Check sheet for the modelled part. Datum: model origin and axes. Units: mm. Round coordinates to 2 decimals unless told otherwise and drop trailing zeros. Order: outer loops, then holes, each group sorted by start corner. A loop starts at its lowest first (then second) coordinate and runs counter-clockwise, first axis right, second up. Notation, with made-up numbers: (71, 15) -> (95, 15) arc R10 cw to (95, 28) -> close; hole circle Ø1 at (31, -5.75). An arc over 180 degrees is marked (long way). Answer in a Markdown table with one row per item.
from build123d import *

# Parameters (mm, degrees)
EXTRUDE1_DEPTH = 0.5
FILLET1_R      = 3
SKETCH3_R      = 13.5
SKETCH3_R_2    = 3.5
SKETCH3_R_3    = 6.25
EXTRUDE2_DEPTH = 0.5
FILLET2_R      = 1


with BuildPart() as part:
    # Sketch1 → Revolve1 (revolve)
    with BuildSketch(Plane(origin=(0, 0, 0), x_dir=(0, 0, -1), z_dir=(1, 0, 0))):
        with BuildLine():
            Line((40, 36), (41.424630354, 28))
            ThreePointArc((41.424630354, 28), (44.158804332, -23.452078799), (0, -50))
            Line((0, -50), (0, 36))
            Line((0, 36), (40, 36))
        make_face()
    revolve(axis=Axis((0, 36, 0), (0, -1, 0)))

    # Sketch2 → Extrude1 (cut)
    with BuildSketch(Plane(origin=(0, 36, 0), x_dir=(1, 0, 0), z_dir=(0, 1, 0))):
        with BuildLine():
            Line((17.811513131, 33), (-17.811513131, 33))
            ThreePointArc((-17.811513131, 33), (-37.5, 0), (-17.811513131, -33))
            Line((-17.811513131, -33), (17.811513131, -33))
            ThreePointArc((17.811513131, -33), (32.20389528, -19.213514223), (37.5, 0))
            ThreePointArc((37.5, 0), (32.20389528, 19.213514223), (17.811513131, 33))
        make_face()
    extrude(amount=-EXTRUDE1_DEPTH, mode=Mode.SUBTRACT)

    # Fillet1
    # the kernel refuses this fillet: 3 mm, written as the material it adds along each edge
    with BuildSketch(Plane(origin=(-21.957294119, 35.5, 33), x_dir=(0, 1.0, -3.3253400033406348e-12), z_dir=(1, 0, 0)), Plane(origin=(21.957294119, 35.5, -33), x_dir=(0, 1.0, 3.3253400033406348e-12), z_dir=(-1, 0, 0))) as fillet1_piece_1:
        with BuildLine():
            CenterArc((3, -1.658312395), FILLET1_R, 146.442690238, 33.557309762)
            Line((0, -1.658312395), (0, 0))
            Line((0, 0), (0.5, 0))
        make_face()
    extrude(amount=43.914588237)
    with BuildSketch(Plane(origin=(0, 35.5, 0), x_dir=(0.37490714563861727, 0, 0.9270623669144945), z_dir=(-0.9270623669144945, 0, 0.37490714563861727))) as fillet1_piece_2:
        with BuildLine():
            CenterArc((35.841687605, 3), FILLET1_R, 270, 33.557309762)
            Line((35.841687605, 0), (37.5, 0))
            Line((37.5, 0), (37.5, 0.5))
        make_face()
    revolve(axis=Axis((0, 35.5, 0), (0, 1, 0)), revolution_arc=135.962852024)
    with BuildSketch(Plane(origin=(0, 35.5, 0), x_dir=(-0.37490714563861693, 0, -0.9270623669144946), z_dir=(0.9270623669144946, 0, -0.37490714563861693))) as fillet1_piece_3:
        with BuildLine():
            CenterArc((35.841687605, 3), FILLET1_R, 270, 33.557309762)
            Line((35.841687605, 0), (37.5, 0))
            Line((37.5, 0), (37.5, 0.5))
        make_face()
    revolve(axis=Axis((0, 35.5, 0), (0, 1, 0)), revolution_arc=135.962852024)

    # Sketch3 → Extrude2 (cut)
    # profile 1 of 10: a face of its own
    with BuildSketch(Plane(origin=(0, 35.5, 0), x_dir=(1, 0, 0), z_dir=(0, 1, 0))):
        with Locations(Location((-17.5, 1.2, 0), (0, 0, 270))):
            Circle(SKETCH3_R)
    # profile 2 of 10: a face of its own
    with BuildSketch(Plane(origin=(0, 35.5, 0), x_dir=(1, 0, 0), z_dir=(0, 1, 0))):
        with Locations(Location((17.5, 1.2, 0), (0, 0, 270))):
            Circle(SKETCH3_R)
        with Locations(Location((17.5, 1.2, 0), (0, 0, 270))):
            Circle(SKETCH3_R_2, mode=Mode.SUBTRACT)
    # profile 3 of 10: a face of its own
    with BuildSketch(Plane(origin=(0, 35.5, 0), x_dir=(1, 0, 0), z_dir=(0, 1, 0))):
        with Locations(Location((0, -20, 0), (0, 0, 270))):
            Circle(SKETCH3_R_3)
    # profile 4 of 10: a face of its own
    with BuildSketch(Plane(origin=(0, 35.5, 0), x_dir=(1, 0, 0), z_dir=(0, 1, 0))):
        with BuildLine():
            Line((-3.75, 24.8), (-1.75, 24.8))
            ThreePointArc((-1.75, 24.8), (-0.75, 23.8), (-1.75, 22.8))
            Line((-1.75, 22.8), (-3.75, 22.8))
            ThreePointArc((-3.75, 22.8), (-4.75, 23.8), (-3.75, 24.8))
        make_face()
    # profile 5 of 10: a face of its own
    with BuildSketch(Plane(origin=(0, 35.5, 0), x_dir=(1, 0, 0), z_dir=(0, 1, 0))):
        with BuildLine():
            Line((-6.5, 27.3), (-4.5, 27.3))
            ThreePointArc((-4.5, 27.3), (-3.5, 26.3), (-4.5, 25.3))
            Line((-4.5, 25.3), (-6.5, 25.3))
            ThreePointArc((-6.5, 25.3), (-7.5, 26.3), (-6.5, 27.3))
        make_face()
    # profile 6 of 10: a face of its own
    with BuildSketch(Plane(origin=(0, 35.5, 0), x_dir=(1, 0, 0), z_dir=(0, 1, 0))):
        with BuildLine():
            Line((-1, 27.3), (1, 27.3))
            ThreePointArc((1, 27.3), (2, 26.3), (1, 25.3))
            Line((1, 25.3), (-1, 25.3))
            ThreePointArc((-1, 25.3), (-2, 26.3), (-1, 27.3))
        make_face()
    # profile 7 of 10: a face of its own
    with BuildSketch(Plane(origin=(0, 35.5, 0), x_dir=(1, 0, 0), z_dir=(0, 1, 0))):
        with BuildLine():
            Line((-3.75, 29.8), (-1.75, 29.8))
            ThreePointArc((-1.75, 29.8), (-0.75, 28.8), (-1.75, 27.8))
            Line((-1.75, 27.8), (-3.75, 27.8))
            ThreePointArc((-3.75, 27.8), (-4.75, 28.8), (-3.75, 29.8))
        make_face()
    # profile 8 of 10: a face of its own
    with BuildSketch(Plane(origin=(0, 35.5, 0), x_dir=(1, 0, 0), z_dir=(0, 1, 0))):
        with BuildLine():
            Line((1.75, 29.8), (3.75, 29.8))
            ThreePointArc((3.75, 29.8), (4.75, 28.8), (3.75, 27.8))
            Line((3.75, 27.8), (1.75, 27.8))
            ThreePointArc((1.75, 27.8), (0.75, 28.8), (1.75, 29.8))
        make_face()
    # profile 9 of 10: a face of its own
    with BuildSketch(Plane(origin=(0, 35.5, 0), x_dir=(1, 0, 0), z_dir=(0, 1, 0))):
        with BuildLine():
            Line((4.5, 27.3), (6.5, 27.3))
            ThreePointArc((6.5, 27.3), (7.5, 26.3), (6.5, 25.3))
            Line((6.5, 25.3), (4.5, 25.3))
            ThreePointArc((4.5, 25.3), (3.5, 26.3), (4.5, 27.3))
        make_face()
    # profile 10 of 10: a face of its own
    with BuildSketch(Plane(origin=(0, 35.5, 0), x_dir=(1, 0, 0), z_dir=(0, 1, 0))):
        with BuildLine():
            Line((1.75, 24.8), (3.75, 24.8))
            ThreePointArc((3.75, 24.8), (4.75, 23.8), (3.75, 22.8))
            Line((3.75, 22.8), (1.75, 22.8))
            ThreePointArc((1.75, 22.8), (0.75, 23.8), (1.75, 24.8))
        make_face()
    extrude(amount=-EXTRUDE2_DEPTH, mode=Mode.SUBTRACT)

    # Fillet2
    # the kernel refuses this fillet: 1 mm, written as the material it adds along each edge
    with BuildSketch(Plane(origin=(0, 35, 20), x_dir=(0, 0, 1), z_dir=(-1, 0, 0))) as fillet2_piece_1:
        with BuildLine():
            CenterArc((5.383974596, 1), FILLET2_R, 270, 60)
            Line((5.383974596, 0), (5.383974596, -0.02))
            Line((5.383974596, -0.02), (6.25, -0.02))
            Line((6.25, -0.02), (6.27, 0))
            ThreePointArc((6.27, 0), (6.27, 0.25), (6.267320508, 0.49))
            Line((6.267320508, 0.49), (6.25, 0.5))
        make_face()
    revolve(axis=Axis((0, 35, 20), (0, 1, 0)))
    with BuildSketch(Plane(origin=(17.5, 35, -1.2), x_dir=(0, 0, 1), z_dir=(-1, 0, 0))) as fillet2_piece_2:
        with BuildLine():
            CenterArc((12.633974596, 1), FILLET2_R, 270, 60)
            Line((12.633974596, 0), (12.633974596, -0.02))
            Line((12.633974596, -0.02), (13.5, -0.02))
            Line((13.5, -0.02), (13.52, 0))
            ThreePointArc((13.52, 0), (13.52, 0.25), (13.517320508, 0.49))
            Line((13.517320508, 0.49), (13.5, 0.5))
        make_face()
    revolve(axis=Axis((17.5, 35, -1.2), (0, 1, 0)))
    with BuildSketch(Plane(origin=(17.5, 35, -1.2), x_dir=(0, 0, 1), z_dir=(-1, 0, 0))) as fillet2_piece_3:
        with BuildLine():
            CenterArc((4.366025404, 1), FILLET2_R, 210, 60)
            Line((3.5, 0.5), (3.482679492, 0.49))
            ThreePointArc((3.482679492, 0.49), (3.48, 0.25), (3.48, 0))
            Line((3.48, 0), (3.5, -0.02))
            Line((3.5, -0.02), (4.366025404, -0.02))
            Line((4.366025404, -0.02), (4.366025404, 0))
        make_face()
    revolve(axis=Axis((17.5, 35, -1.2), (0, 1, 0)))
    with BuildSketch(Plane(origin=(-17.5, 35, -1.2), x_dir=(0, 0, 1), z_dir=(-1, 0, 0))) as fillet2_piece_4:
        with BuildLine():
            CenterArc((12.633974596, 1), FILLET2_R, 270, 60)
            Line((12.633974596, 0), (12.633974596, -0.02))
            Line((12.633974596, -0.02), (13.5, -0.02))
            Line((13.5, -0.02), (13.52, 0))
            ThreePointArc((13.52, 0), (13.52, 0.25), (13.517320508, 0.49))
            Line((13.517320508, 0.49), (13.5, 0.5))
        make_face()
    revolve(axis=Axis((-17.5, 35, -1.2), (0, 1, 0)))


solid = part.part
Item 1: Scan lines: line 1 (X direction, y = 20.5, z = 15); line 2 (Y direction, x = 23.5, z = 20); line 3 (X direction, y = 10, z = -23). Record each from-to range of solid material in increasing order. Write a range as [from, to].
Result sheet:
| item | result |
|---|---|
| line 1 | x = [-43.07, 43.07] |
| line 2 | y = [-39.34, 35.5] |
| line 3 | x = [-43.26, 43.26] |
Item 2: Cross-section at A-A (y = 1.5). Record the boundary of the cut face in (x, z).
Result sheet:
| item | result |
|---|---|
| outline | circle Ø99.95 at (0, 0) |
Item 3: Cross-section at B-B (x = 44.5). Record the boundary of the cut face in (y, z), and give its area (3 significant figures).
Result sheet:
| item | result |
|---|---|
| outline | circle Ø45.6 at (0, 0) |
| area | 1,630 mm^2 |
Item 4: Mould release check, pull along Z, two halves, no side actions. Record for faces 1 (the flat face through (18, 35, 4)), 2 (the conical face through (-39.136, 35.5, 8.691)), 3 (the flat face through (0, 36, 35)): pulls with the +Z half, pulls with the -Z half, needs draft (parallel to the pull), parting line crosses it, or undercut.
Result sheet:
| item | result |
|---|---|
| face 1 | undercut |
| face 2 | parting line crosses it |
| face 3 | needs draft |
Item 5: Depth check by flat-ended pin: P1, Ø12, axis at y = -29, z = 30.5, coming from the -X side; P2, Ø8, axis at x = 17, y = -2, coming from the +Z side; P3, Ø2, axis at x = 16, z = -1, coming from the +Y side. Enter the tip coordinate at first touch or a pass-through.
Result sheet:
| item | result |
|---|---|
| P1 | stops at x = -34.61 |
| P2 | stops at z = 48.25 |
| P3 | stops at y = 35.5 |
